Design review of the part built by this model. Coordinates are the model's own, in mm. A direction names the side the tool comes from. Coordinates: 2 decimals unless noted, no trailing zeros. One line per question, with ' | ' between items.
from build123d import *

# Parameters (mm, degrees)
SKETCH_1_W             = 23.5
SKETCH_1_H             = 12
EXTRUDE_1_DEPTH        = 601
HOLE_WIZARD_M6_1_D     = 5
HOLE_WIZARD_M6_1_DEPTH = 15
HOLE_WIZARD_M6_1_TIP   = 1.502151548
HOLE_WIZARD_M6_2_D     = 5
HOLE_WIZARD_M6_2_DEPTH = 15
HOLE_WIZARD_M6_2_TIP   = 1.502151548
SKETCH_6_R             = 5.05
CUT_EXTRUDE_1_DEPTH    = 602.935212461
HOLE_WIZARD_M4_1_D     = 3.3
HOLE_WIZARD_M4_1_DEPTH = 10.1
HOLE_WIZARD_M4_1_TIP   = 0.991420021
SKETCH_9_R             = 4.5
CUT_EXTRUDE_2_DEPTH    = 602.935212461
HOLE_WIZARD_M4_2_D     = 3.3
HOLE_WIZARD_M4_2_DEPTH = 10.1
HOLE_WIZARD_M4_2_TIP   = 0.991420021


with BuildPart() as part:
    # 草图1 → 凸台-拉伸1 (new, symmetric)
    with BuildSketch(Plane(origin=(0, 0, 0), x_dir=(0, 0, -1), z_dir=(1, 0, 0))):
        with BuildLine():
            Line((-14, 15), (-11.5, 15))
            Line((-11.5, 15), (-11.5, 13.5))
            Line((-11.5, 13.5), (-11.4, 13.5))
            ThreePointArc((-11.4, 13.5), (-11.117157288, 13.382842712), (-11, 13.1))
            Line((-11, 13.1), (-11, 12))
            Line((-11, 12), (-9.5, 12))
            Line((-9.5, 12), (-9.5, 15))
            Line((-9.5, 15), (-8, 15))
            Line((-8, 15), (-8, 12.5))
            Line((-8, 12.5), (-5, 12.5))
            Line((-5, 12.5), (-5, 15))
            Line((-5, 15), (5, 15))
            Line((5, 15), (5, 12.5))
            Line((5, 12.5), (8, 12.5))
            Line((8, 12.5), (8, 15))
            Line((8, 15), (9.5, 15))
            Line((9.5, 15), (9.5, 12))
            Line((9.5, 12), (11, 12))
            Line((11, 12), (11, 13.1))
            ThreePointArc((11, 13.1), (11.117157288, 13.382842712), (11.4, 13.5))
            Line((11.4, 13.5), (11.5, 13.5))
            Line((11.5, 13.5), (11.5, 15))
            Line((11.5, 15), (14, 15))
            ThreePointArc((14, 15), (14.707106781, 14.707106781), (15, 14))
            Line((15, 14), (15, 8))
            Line((15, 8), (12.5, 8))
            Line((12.5, 8), (12.5, 5))
            Line((12.5, 5), (15, 5))
            Line((15, 5), (15, -5))
            Line((15, -5), (12.5, -5))
            Line((12.5, -5), (12.5, -8))
            Line((12.5, -8), (15, -8))
            Line((15, -8), (15, -14))
            ThreePointArc((15, -14), (14.707106781, -14.707106781), (14, -15))
            Line((14, -15), (11.5, -15))
            Line((11.5, -15), (11.5, -13.5))
            Line((11.5, -13.5), (11.4, -13.5))
            ThreePointArc((11.4, -13.5), (11.117157288, -13.382842712), (11, -13.1))
            Line((11, -13.1), (11, -12))
            Line((11, -12), (9.5, -12))
            Line((9.5, -12), (9.5, -15))
            Line((9.5, -15), (8, -15))
            Line((8, -15), (8, -12.5))
            Line((8, -12.5), (5, -12.5))
            Line((5, -12.5), (5, -15))
            Line((5, -15), (-5, -15))
            Line((-5, -15), (-5, -12.5))
            Line((-5, -12.5), (-8, -12.5))
            Line((-8, -12.5), (-8, -15))
            Line((-8, -15), (-9.5, -15))
            Line((-9.5, -15), (-9.5, -12))
            Line((-9.5, -12), (-11, -12))
            Line((-11, -12), (-11, -13.1))
            ThreePointArc((-11, -13.1), (-11.117157288, -13.382842712), (-11.4, -13.5))
            Line((-11.4, -13.5), (-11.5, -13.5))
            Line((-11.5, -13.5), (-11.5, -15))
            Line((-11.5, -15), (-14, -15))
            ThreePointArc((-14, -15), (-14.707106781, -14.707106781), (-15, -14))
            Line((-15, -14), (-15, 14))
            ThreePointArc((-15, 14), (-14.707106781, 14.707106781), (-14, 15))
        make_face()
        with BuildLine():
            Line((12, -10.5), (12, -8.5))
            ThreePointArc((12, -8.5), (11.853553391, -8.146446609), (11.5, -8))
            Line((11.5, -8), (-11.5, -8))
            ThreePointArc((-11.5, -8), (-11.853553391, -8.146446609), (-12, -8.5))
            Line((-12, -8.5), (-12, -10.5))
            ThreePointArc((-12, -10.5), (-11.853553391, -10.853553391), (-11.5, -11))
            Line((-11.5, -11), (11.5, -11))
            ThreePointArc((11.5, -11), (11.853553391, -10.853553391), (12, -10.5))
        make_face(mode=Mode.SUBTRACT)
        with BuildLine():
            Line((-11.5, 11), (11.5, 11))
            ThreePointArc((11.5, 11), (11.853553391, 10.853553391), (12, 10.5))
            Line((12, 10.5), (12, 8.5))
            ThreePointArc((12, 8.5), (11.853553391, 8.146446609), (11.5, 8))
            Line((11.5, 8), (-11.5, 8))
            ThreePointArc((-11.5, 8), (-11.853553391, 8.146446609), (-12, 8.5))
            Line((-12, 8.5), (-12, 10.5))
            ThreePointArc((-12, 10.5), (-11.853553391, 10.853553391), (-11.5, 11))
        make_face(mode=Mode.SUBTRACT)
        Rectangle(SKETCH_1_W, SKETCH_1_H, mode=Mode.SUBTRACT)
    extrude(amount=EXTRUDE_1_DEPTH, both=True)

    # M6 螺纹孔1
    with Locations(Plane(origin=(0, 0, -15), x_dir=(-1, 0, 0), z_dir=(0, 0, -1))):
        with Locations((-551, 0), (-536, 0), (536, 0), (551, 0)):
            Hole(HOLE_WIZARD_M6_1_D / 2, depth=HOLE_WIZARD_M6_1_DEPTH)
            with Locations((0, 0, -(HOLE_WIZARD_M6_1_DEPTH + HOLE_WIZARD_M6_1_TIP / 2))):  # 118° drill point
                Cone(0, HOLE_WIZARD_M6_1_D / 2, HOLE_WIZARD_M6_1_TIP, mode=Mode.SUBTRACT)

    # M6 螺纹孔2
    with Locations(Plane.XZ.offset(15)):
        with Locations((551, 0), (536, 0), (299, 0), (284, 0), (214, 0), (199, 0), (-536, 0), (-551, 0)):
            Hole(HOLE_WIZARD_M6_2_D / 2, depth=HOLE_WIZARD_M6_2_DEPTH)
            with Locations((0, 0, -(HOLE_WIZARD_M6_2_DEPTH + HOLE_WIZARD_M6_2_TIP / 2))):  # 118° drill point
                Cone(0, HOLE_WIZARD_M6_2_D / 2, HOLE_WIZARD_M6_2_TIP, mode=Mode.SUBTRACT)

    # 草图6 → 切除-拉伸1 (cut, through all)
    with BuildSketch(Plane.XZ.offset(15)):
        with Locations(Location((-586, 0, 0), (0, 0, 90))):
            Circle(SKETCH_6_R)
        with Locations(Location((-88, 0, 0), (0, 0, 90))):
            Circle(SKETCH_6_R)
    extrude(amount=-CUT_EXTRUDE_1_DEPTH, mode=Mode.SUBTRACT)

    # M4 螺纹孔1
    with Locations(Plane.XZ.offset(15)):
        with Locations((-489, 0), (-329, 0), (-169, 0), (-9, 0), (151, 0)):
            Hole(HOLE_WIZARD_M4_1_D / 2, depth=HOLE_WIZARD_M4_1_DEPTH)
            with Locations((0, 0, -(HOLE_WIZARD_M4_1_DEPTH + HOLE_WIZARD_M4_1_TIP / 2))):  # 118° drill point
                Cone(0, HOLE_WIZARD_M4_1_D / 2, HOLE_WIZARD_M4_1_TIP, mode=Mode.SUBTRACT)

    # 草图9 → 切除-拉伸2 (cut, through all)
    with BuildSketch(Plane.XY.offset(15)):
        with Locations((501, 0)):
            Circle(SKETCH_9_R)
        with Locations((-501, 0)):
            Circle(SKETCH_9_R)
    extrude(amount=-CUT_EXTRUDE_2_DEPTH, mode=Mode.SUBTRACT)

    # M4 螺纹孔2
    with Locations(Plane(origin=(0, 0, -15), x_dir=(-1, 0, 0), z_dir=(0, 0, -1))):
        with Locations((-454, 0), (-259, 0), (-64, 0), (131, 0), (326, 0)):
            Hole(HOLE_WIZARD_M4_2_D / 2, depth=HOLE_WIZARD_M4_2_DEPTH)
            with Locations((0, 0, -(HOLE_WIZARD_M4_2_DEPTH + HOLE_WIZARD_M4_2_TIP / 2))):  # 118° drill point
                Cone(0, HOLE_WIZARD_M4_2_D / 2, HOLE_WIZARD_M4_2_TIP, mode=Mode.SUBTRACT)


solid = part.part
1. Tool access review of faces 1 (the face through (8, 6, 0)), 2 (the face through (-601, 7, 0)): name each direction out of +Z, -Z, +X, -X, +Y, -Y from which nothing blocks a thin tool from reaching the whole face with its end or side.
Answer sheet:
face 1: +X, -X | face 2: +Z, -Z, -X, +Y, -Y
2. Insertion check: pin 1 Ø2 at (x, z) = (-9, 0) entering from -Y; pin 2 Ø1.6 at (x, z) = (-245, 10.5) entering from +Y. Each pin has a flat end and moves straight along its axis. Give the tip position at first contact, or say it passes through.
Answer sheet:
pin 1: y = 6 | pin 2: y = 13.49
3. Draft analysis for pull direction Y (two halves, no side actions). For faces 3 (the face through (8, -8, 0)), 4 (the face through (8, -6, 0)), 5 (the face through (8, 0, 15)), state which applies: pulls with the +Y half, pulls with the -Y half, needs draft (parallel to the pull), parting line crosses it, or undercut.
Answer sheet:
face 3: undercut | face 4: undercut | face 5: needs draft
4. To check wall thickness, follow line 1 along Z through (x, y) = (-394, -12.75); line 2 along Y through (x, z) = (-400, 3); line 3 along Y through (x, z) = (-165.5, -12.75). State the ranges of each line that lie inside material, in increasing order. Write a range as [from, to].
Answer sheet:
line 1: [-15, -11], [-9.5, -8], [-5, 5], [8, 9.5], [11, 15] | line 2: [-15, -11], [-8, -6], [6, 8], [11, 15] | line 3: [-15, -8], [-5, 5], [8, 15]
5. Take a section at A-A (x = 363). Count the separate pieces of the cut face and the enclosed holes in it, then the cut area to 3 significant figures.
Answer sheet:
separate pieces: 1 | enclosed holes: 3 | area: 407 mm^2
